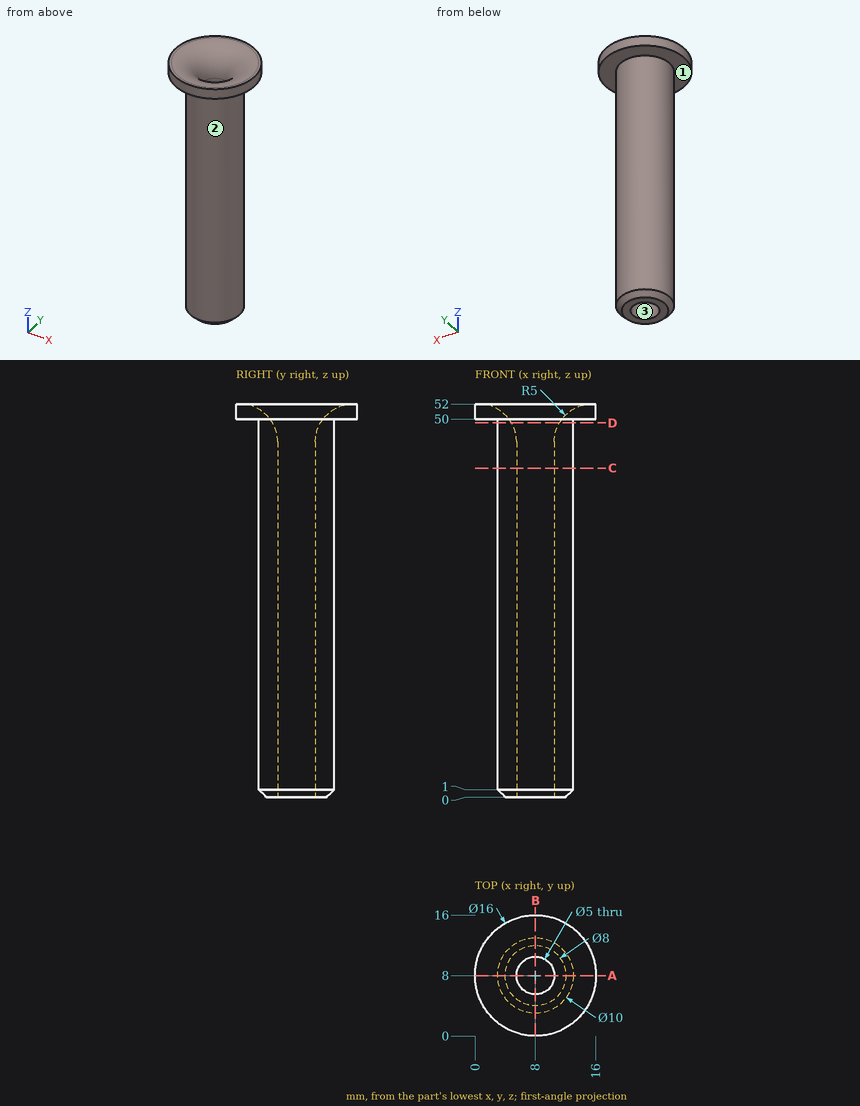
Could you check a few things on this drawing? It's one solid part, dimensions in mm from its lowest x, y, z. Coordinates: 2 decimals unless noted, no trailing zeros. Order: outer loops, then holes, each group sorted by start corner. A loop starts at its lowest first (then second) coordinate and runs counter-clockwise, first axis right, second up.
1) Imagine slicing it at C-C on z = 43.5. List the corners of the cut face in (x, y) for me, and give its area (3 significant figures).
2) Imagine slicing it at D-D on z = 49.5. List the corners of the cut face in (x, y) for me.
3) I need wall thicknesses on line 1 (X direction, y = 8, z = 29); line 2 (Y direction, x = 9, z = 34). Which ranges of each line are inside material? Lowest first, please.
4) Will these pins go through, and if not, where does the flat tip stop? pin 1 (5 mm diameter, centred on y = 5, z = 28.5, fed in from +X); pin 2 (8 mm diameter, centred on x = 8, y = 8, fed in from +Z); pin 3 (1.5 mm diameter, centred on x = 5.5, z = 25, fed in from -Y); pin 4 (1.5 mm diameter, centred on y = 14, z = 39, fed in from +X).
5) Imagine slicing it at A-A on y = 8. List the corners of the cut face in (x, z) for me.
6) We'd pull the mould along Y, two halves only. Please class the marked faces 1, 2 and 3: +Y half, -Y half, draft (parallel to the pull), parting line (faces both ways), or undercut.
Response values:
1. outline: circle Ø10 at (8, 8); hole circle Ø5 at (8, 8)
1. area: 58.9 mm2
2. outline: circle Ø10 at (8, 8); hole circle Ø6.34 at (8, 8)
3. line 1: x = 3 to 5.5, 10.5 to 13
3. line 2: y = 3.1 to 5.71, 10.29 to 12.9
4. pin 1: stops at x = 12.97
4. pin 2: stops at z = 50.57
4. pin 3: stops at y = 3.32
4. pin 4: passes through
5. outline: (0, 50) - (3, 50) - (3, 1) - (4, 0) - (5.5, 0) - (5.5, 47) arc R5 ccw to (0.5, 52) - (0, 52) - close; (10.5, 0) - (12, 0) - (13, 1) - (13, 50) - (16, 50) - (16, 52) - (15.5, 52) arc R5 ccw to (10.5, 47) - close
6. face 1: draft
6. face 2: parting line
6. face 3: undercut
